Here's how the part is built. I have some questions about the finished solid (model axes, mm). Face numbers are marked on the shaded views. Round coordinates to 2 decimals unless told otherwise and drop trailing zeros. Loops run counter-clockwise (first coordinate to the right, second up) from the corner with the lowest first, then second, coordinate; pieces in that order, holes last. Notation, with made-up numbers: (-29.75, 58.25) - (-22.75, 58.25) arc R28 ccw to (-22.75, 93.25) - close; hole circle Ø7 at (33.5, 26). An arc over 180 degrees is marked (long way). Answer as a JSON object with one key per item and string values. Group by question number.
1) I want a section at C-C, the plane z = -0.65. Please give me the cut outline in (x, y).
2) If I drill on line 1 along Y through (x, z) = (0, 0.35); line 2 along Y through (x, z) = (0, -0.3); line 3 along Z through (x, y) = (-1.5, -3.5), over which ranges is the centre line in solid material (lowest first)? Write a range as [from, to].
3) I want a section at A-A, the plane x = 0. Please give me the cut outline in (y, z).
4) I want a section at B-B, the plane y = 0. Please give me the cut outline in (x, z), then the cut area to 3 significant figures.
5) Will these pins go through, and if not, where does the flat tip stop? P1, Ø1.8, axis at x = 0, y = -6, coming from the +Z side; P2, Ø3, axis at x = 5, y = -7, coming from the -Z side.
6) I want a section at D-D, the plane z = 1.55. Please give me the cut outline in (x, y), then the cut area to 3 significant figures.
7) If we mould it in two halves opening along X, with no side actions, what happens to the marked faces 1, 2 and 3? For each: pulls with the +X half, pulls with the -X half, needs draft (parallel to the pull), parting line crosses it, or undercut.
from build123d import *

# Parameters (mm, degrees)
F0_R           = 9
F0_R_2         = 3.5
F0_R_3         = 2
F1_DEPTH       = 2
F2_DEPTH       = 1
F4_D           = 2
F4_CSINK_D     = 4
F4_CSINK_ANGLE = 90


with BuildPart() as f1:
    # F0 (on Top) → F1 (new body)
    with BuildSketch(Plane.XY):
        Circle(F0_R)
        Circle(F0_R_2, mode=Mode.SUBTRACT)
        Circle(F0_R_2)
        Circle(F0_R_3, mode=Mode.SUBTRACT)
    extrude(amount=F1_DEPTH)

    # F0 (on Top) → F2 (join)
    with BuildSketch(Plane.XY):
        Circle(F0_R_2)
        Circle(F0_R_3, mode=Mode.SUBTRACT)
    extrude(amount=-F2_DEPTH)

    # F4 (through all)
    with Locations(Plane.XY.offset(2)):
        with Locations((0, 6), (0, -6)):
            CounterSinkHole(F4_D / 2, F4_CSINK_D / 2, counter_sink_angle=F4_CSINK_ANGLE)


solid = f1.part
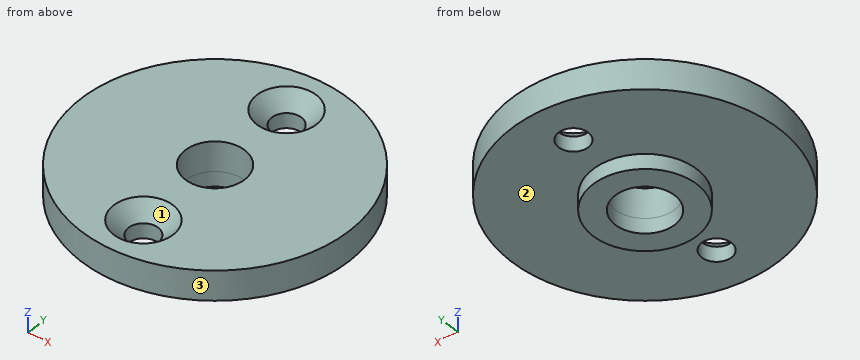
Outcome:
{
 "1": {"outline": "circle Ø7 at (0, 0); hole circle Ø4 at (0, 0)"},
 "2": {"line 1": "[-9, -7], [-5, -2], [2, 5], [7, 9]", "line 2": "[-3.5, -2], [2, 3.5]", "line 3": "[0, 2]"},
 "3": {"outline": "(-9, 0) - (-7, 0) - (-7, 1) - (-8, 2) - (-9, 2) - close; (-5, 0) - (-3.5, 0) - (-3.5, -1) - (-2, -1) - (-2, 2) - (-4, 2) - (-5, 1) - close; (2, -1) - (3.5, -1) - (3.5, 0) - (5, 0) - (5, 1) - (4, 2) - (2, 2) - close; (7, 0) - (9, 0) - (9, 2) - (8, 2) - (7, 1) - close"},
 "4": {"outline": "(-9, 0) - (-3.5, 0) - (-3.5, -1) - (-2, -1) - (-2, 2) - (-9, 2) - close; (2, -1) - (3.5, -1) - (3.5, 0) - (9, 0) - (9, 2) - (2, 2) - close", "area": "31.0 mm^2"},
 "5": {"P1": "through", "P2": "z = 0"},
 "6": {"outline": "circle Ø18 at (0, 0); hole circle Ø4 at (0, 0); hole circle Ø3.1 at (0, -6); hole circle Ø3.1 at (0, 6)", "area": "227 mm^2"},
 "7": {"face 1": "undercut", "face 2": "needs draft", "face 3": "parting line crosses it"}
}
